For this review, take the finished solid that the model builds, in its own axes (mm). A direction names the side the tool comes from. Round coordinates to 2 decimals unless told otherwise and drop trailing zeros. Order: outer loops, then holes, each group sorted by start corner. A loop starts at its lowest first (then second) coordinate and runs counter-clockwise, first axis right, second up. Notation, with made-up numbers: M 42,-28.75 L 66,-28.75 A25 ccw 66,-7.75 Z; hole C -17,-0.5 d10. An arc over 180 degrees is marked long. Answer as a JSON object with one key per item and string values.
from build123d import *

# Parameters (mm, degrees)
SKETCH1_W           = 40
SKETCH1_H           = 30
BOSS_EXTRUDE1_DEPTH = 23
SKETCH2_W           = 19.900467999
SKETCH2_H           = 6.66107141
CUT_EXTRUDE1_DEPTH  = 19
SKETCH3_R           = 2
CUT_EXTRUDE2_DEPTH  = 19
BOSS_EXTRUDE2_DEPTH = 8


with BuildPart() as part:
    # Sketch1 → Boss-Extrude1 (new body)
    with BuildSketch(Plane.XY):
        Rectangle(SKETCH1_W, SKETCH1_H)
    extrude(amount=BOSS_EXTRUDE1_DEPTH)

    # Sketch2 → Cut-Extrude1 (cut)
    with BuildSketch(Plane.XY.offset(23)):
        Polygon((-3.475341605, 7.20854355), (-3.475341605, -3.599460948), (16.425126394, -3.599460948), (16.425126394, 7.20854355), (11.005248415, 11.99820316), (1.944536374, 11.99820316), align=None)
        with Locations((6.474892394, -9.412383513)):
            Rectangle(SKETCH2_W, SKETCH2_H)
    extrude(amount=-CUT_EXTRUDE1_DEPTH, mode=Mode.SUBTRACT)

    # Sketch3 → Cut-Extrude2 (cut)
    with BuildSketch(Plane(origin=(0, -12.742919218, 0), x_dir=(1, 0, 0), z_dir=(0, 1, 0))):
        with Locations((6.578325181, -13)):
            Circle(SKETCH3_R)
    extrude(amount=-CUT_EXTRUDE2_DEPTH, mode=Mode.SUBTRACT)

    # Sketch4 → Boss-Extrude2 (add)
    with BuildSketch(Plane.ZY.offset(17)):
        with BuildLine():
            Line((23, 12), (23.778195764, 12))
            ThreePointArc((23.778195764, 12), (24.486476148, -0.348459209), (28.637102986, -12))
            Line((28.637102986, -12), (23, -12))
            Line((23, -12), (23, 12))
        make_face()
    extrude(amount=-BOSS_EXTRUDE2_DEPTH)


solid = part.part
1) Add section C-C on x = 6.5. State the section outline as (y, z) points, and give its area (3 significant figures).
Geometry check:
{"outline": "M -15,0 L 15,0 L 15,23 L 12,23 L 12,4 L -3.6,4 L -3.6,23 L -6.08,23 L -6.08,4 L -12.74,4 L -12.74,11 L -15,11 Z; M -15,15 L -12.74,15 L -12.74,23 L -15,23 Z", "area": "258 mm²"}
2) Mouldability with a two-part tool opening along X and no side actions: class faces 4 (the flat face through (-9, -4, 25)), 5 (the flat face through (-0.727, 9.637, 13.633)), 6 (the flat face through (-17, -4, 25)) as +X half, -X half, draft (parallel to the pull), parting line (faces both ways), or undercut.
Geometry check:
{"face 4": "+X half", "face 5": "undercut", "face 6": "-X half"}
3) Insertion check: P1, Ø1.5, axis at x = 6, y = -4.5, coming from the +Z side; P2, Ø2, axis at x = 4.5, y = -8, coming from the +Z side; P3, Ø3, axis at x = 6.58, z = 13, coming from the -Y side. Each pin has a flat end and moves straight along its axis. Give the tip position at first contact, or say it passes through.
Geometry check:
{"P1": "stops at z = 23", "P2": "stops at z = 4", "P3": "stops at y = -6.08"}
4) Add section D-D on x = -3. State the section outline as (y, z) points, and give its area (3 significant figures).
Geometry check:
{"outline": "M -15,0 L 15,0 L 15,23 L 7.63,23 L 7.63,4 L -3.6,4 L -3.6,23 L -6.08,23 L -6.08,4 L -12.74,4 L -12.74,23 L -15,23 Z", "area": "350 mm²"}
5) For L1, parallel to Y at x = 11, z = 21.5; L2, parallel to X at y = -7, z = 4.25; L3, parallel to X at y = -13.95, z = 13, list the stretches that pass through material, from the lowest coordinate up.
Geometry check:
{"L1": "y = -15 to -12.74, -6.08 to -3.6, 12 to 15", "L2": "x = -20 to -3.48, 16.43 to 20", "L3": "x = -20 to 4.58, 8.58 to 20"}
6) Machinability: for faces 1 (the flat face through (-13, -12, 26)), 2 (the flat face through (7, 11.998, 14)), 3 (the cylindrical face through (7.65, -13.86, 11.31)), which of the approach directions +Z, -Z, +X, -X, +Y, -Y give a long, thin tool a straight path to every point of the face, cutting with its end or side? Answer none if there is none.
Geometry check:
{"face 1": "+Z, +X, -X, -Y", "face 2": "+Z", "face 3": "-Y"}
7) Add section B-B on z = 13. State the section outline as (x, y) points.
Geometry check:
{"outline": "M -20,-15 L 4.58,-15 L 4.58,-12.74 L -3.48,-12.74 L -3.48,-6.08 L 16.43,-6.08 L 16.43,-12.74 L 8.58,-12.74 L 8.58,-15 L 20,-15 L 20,15 L -20,15 Z; hole M -3.48,-3.6 L 16.43,-3.6 L 16.43,7.21 L 11.01,12 L 1.94,12 L -3.48,7.21 Z"}
8) Add section A-A on z = 6.5. State the section outline as (x, y) points.
Geometry check:
{"outline": "M -20,-15 L 20,-15 L 20,15 L -20,15 Z; hole M -3.48,-12.74 L 16.43,-12.74 L 16.43,-6.08 L -3.48,-6.08 Z; hole M -3.48,-3.6 L 16.43,-3.6 L 16.43,7.21 L 11.01,12 L 1.94,12 L -3.48,7.21 Z"}
